Can you work these out from the drawing? Everything is in mm from the part's minimum corner. A direction names the side the tool comes from. Give positions to 0.01 mm unless a question says otherwise; leave off trailing zeros. Order: outer loops, then holes, each group sorted by start corner. A loop starts at its lowest first (then second) coordinate and runs counter-clockwise, first axis right, second up. Notation, with made-up numbers: (26, 74.5) - (75, 74.5) arc R26 ccw to (75, 90.5) - close; hole circle Ø5 at (-14.5, 29.5). An arc over 180 degrees is marked (long way). Answer as a JSON object with one key per item and string values.
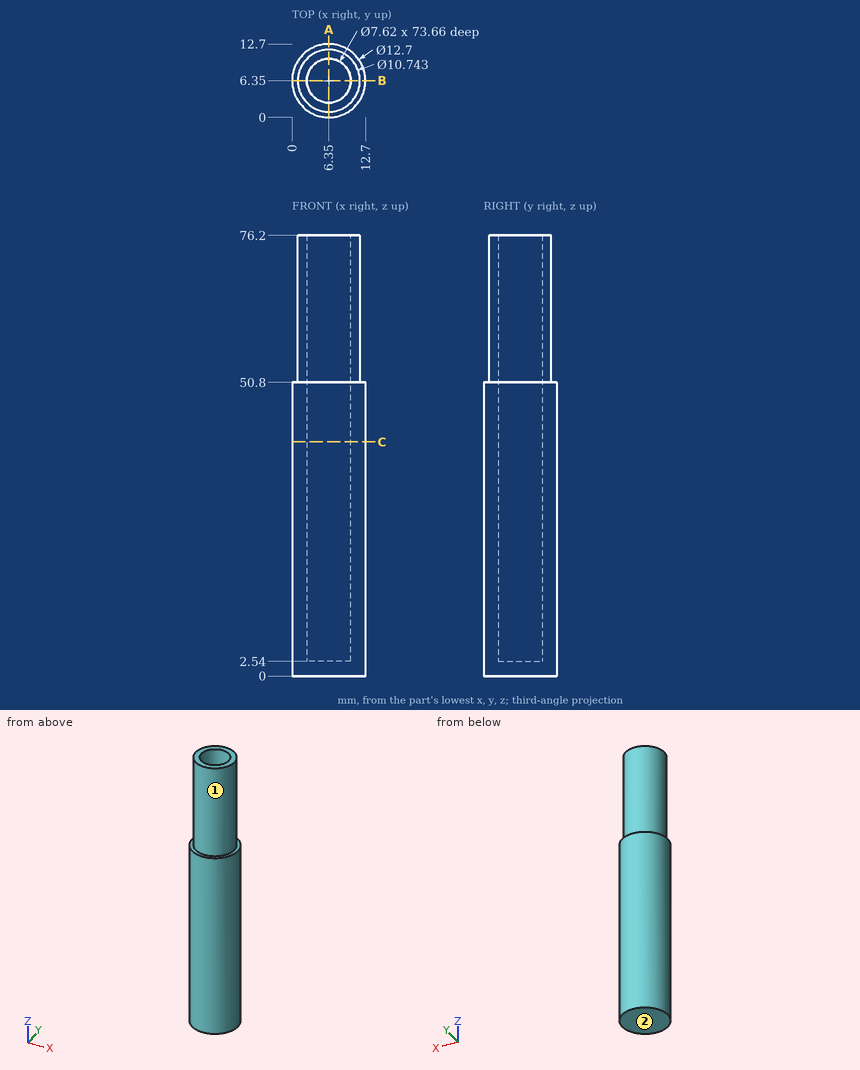
Q1. I need wall thicknesses on L1, parallel to Y at x = 6.35, z = 38.5; L2, parallel to Y at x = 5.75, z = 25. Which ranges of each line are inside material? Lowest first, please.
Recorded:
{"L1": "y = 0 to 2.54, 10.16 to 12.7", "L2": "y = 0.03 to 2.59, 10.11 to 12.67"}
Q2. Which directions (+Z, -Z, +X, -X, +Y, -Y) give clear straight access to the entire face, cutting with the end or side of a thin tool? Please do the marked faces 1 and 2.
Recorded:
{"face 1": "+Z", "face 2": "-Z, +X, -X, +Y, -Y"}
Q3. If we section it at C-C, the plane z = 40.5: Please give me the cut outline in (x, y).
Recorded:
{"outline": "circle Ø12.7 at (6.35, 6.35); hole circle Ø7.62 at (6.35, 6.35)"}
Q4. If we section it at A-A, the plane x = 6.35: Please give me the cut outline in (y, z).
Recorded:
{"outline": "(0, 0) - (12.7, 0) - (12.7, 50.8) - (11.72, 50.8) - (11.72, 76.2) - (10.16, 76.2) - (10.16, 2.54) - (2.54, 2.54) - (2.54, 76.2) - (0.98, 76.2) - (0.98, 50.8) - (0, 50.8) - close"}
Q5. I'm going to push flat-ended pins straight in: pin 1 Ø2 at (x, y) = (4.5, 4.5) entering from +Z; pin 2 Ø3 at (x, z) = (11, 16) entering from +Y. Where does each tip first touch, or does it pass through?
Recorded:
{"pin 1": "stops at z = 2.54", "pin 2": "stops at y = 11.86"}
